The figure shows three views and two pictorial views of one solid part (mm, origin at its lowest corner). Answer the questions. A direction names the side the tool comes from. Round coordinates to 2 decimals unless told otherwise and drop trailing zeros. Write each loop counter-clockwise with the first axis right and the second up, starting at its lowest first coordinate (ties: lowest second). Pieces come first, ordered by that corner, then holes. Notation, with made-up numbers: M 66.25,-36.5 L 123.25,-36.5 A14 cw 123.25,-14.5 Z; hole C 38,-27 d5. An arc over 180 degrees is marked long. Use one line per item in the form item = value. Start each with the question number.
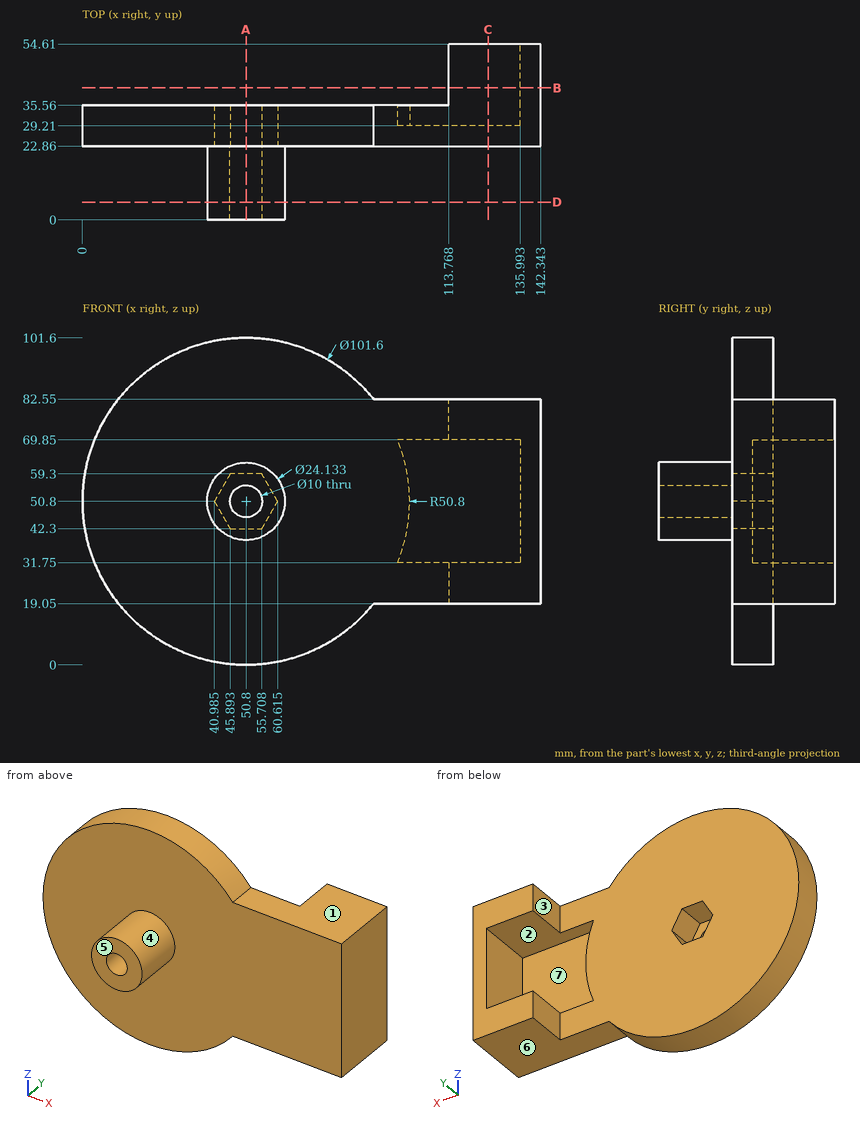
Q1. A tool of negligible diameter and unlimited length cuts with its end or side. For the marked faces 1, 2, 3 and 4, from which of +Z, -Z, +X, -X, +Y, -Y can it reach the whole face along a straight path? Write none if from no direction.
Q2. Straight lines are drawn through the part: line 1 (Z direction, x = 50.8, y = 17.5); line 2 (Z direction, x = 50, y = 16) (1 decimal). For each, find the intervals that lie inside material, in ascending order. Write a range as [from, to].
Q3. Find section D-D on y = 5.5. Write down the section's boundary in (x, z).
Q4. Find section A-A on x = 50.8. Write down the section's boundary in (y, z).
Q5. Find section B-B on y = 41. Write down the section's boundary in (x, z), and give its area (3 significant figures).
Q6. Find section C-C on x = 126. Write down the section's boundary in (y, z), and give its area (3 significant figures).
Q7. For a pull along Z with two mould halves and no side action, classify the marked faces 5, 6 and 7 as +Z half, -Z half, draft (parallel to the pull), parting line (faces both ways), or undercut.
Q8. Each of these flat-tipped pins is pushed along its axis until it touches: pin 1 Ø10 at (y, z) = (49.5, 77.5) entering from -X; pin 2 Ø4 at (x, z) = (67, 73.5) entering from +Y; pin 3 Ø2 at (x, y) = (107.5, 32) entering from -Z. Where does it stop, or does it pass through?
Response:
q1.face_1 = +Z, +X, +Y, -Y
q1.face_2 = +Y
q1.face_3 = +Z, -Z, -X, +Y
q1.face_4 = -Y
q2.line_1 = [38.73, 45.8], [55.8, 62.87]
q2.line_2 = [38.8, 45.9], [55.7, 62.8]
q3.outline = C 50.8,50.8 d24.13; hole C 50.8,50.8 d10
q4.outline = M 0,38.73 L 22.86,38.73 L 22.86,0 L 35.56,0 L 35.56,42.3 L 22.86,42.3 L 22.86,45.8 L 0,45.8 Z; M 0,55.8 L 22.86,55.8 L 22.86,59.3 L 35.56,59.3 L 35.56,101.6 L 22.86,101.6 L 22.86,62.87 L 0,62.87 Z
q5.outline = M 113.77,19.05 L 142.34,19.05 L 142.34,82.55 L 113.77,82.55 L 113.77,69.85 L 135.99,69.85 L 135.99,31.75 L 113.77,31.75 Z
q5.area = 968 mm²
q6.outline = M 22.86,19.05 L 54.61,19.05 L 54.61,31.75 L 29.21,31.75 L 29.21,69.85 L 54.61,69.85 L 54.61,82.55 L 22.86,82.55 Z
q6.area = 1,050 mm²
q7.face_5 = draft
q7.face_6 = -Z half
q7.face_7 = undercut
q8.pin_1 = 113.77
q8.pin_2 = 35.56
q8.pin_3 = 19.05
